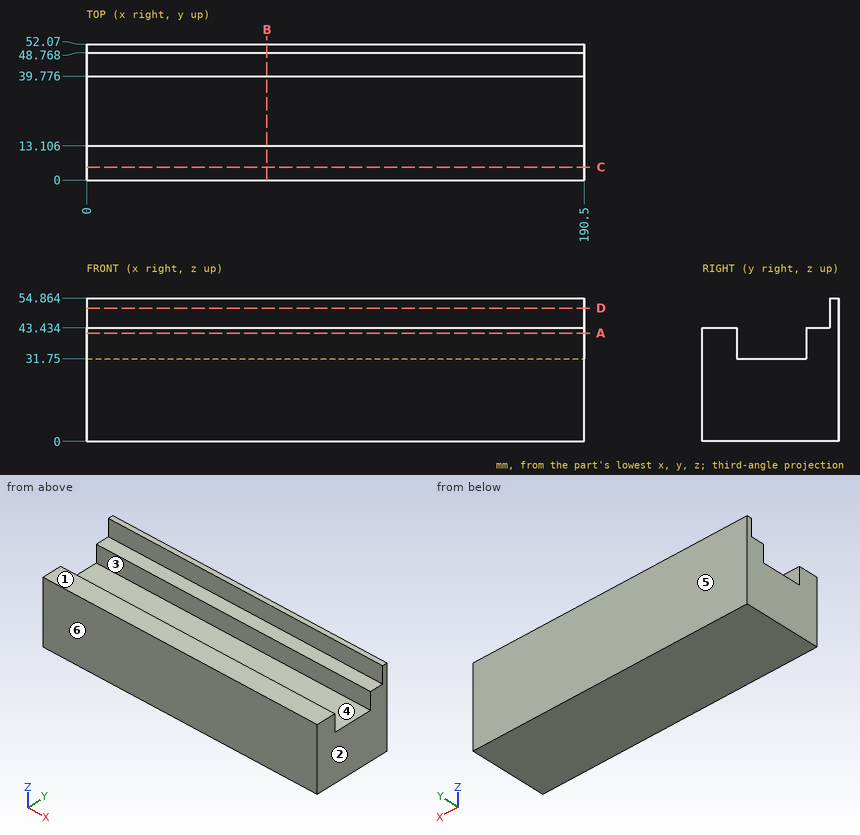
Geometry check sheet. Reference: drawing and pictorial views, mm from the part's lowest x, y, z. A direction names the side the tool comes from. Round coordinates to 2 decimals unless told otherwise and drop trailing zeros. Loops run counter-clockwise (first coordinate to the right, second up) from the corner with the lowest first, then second, coordinate; pieces in that order, holes last. Notation, with made-up numbers: M 36.25,50 L 86.25,50 A7 ccw 86.25,63 Z; hole C 81.5,1 d2. An arc over 180 degrees is marked long. Return JSON: item names as keys, results as strings. Group by question number.
(1) Section check C-C, the plane y = 5. Enter the section's corners in (x, z), and give its area (3 significant figures).
(2) Section check B-B, the plane x = 69. Enter the section's corners in (y, z).
(3) Section check A-A, the plane z = 41.5. Enter the section's corners in (x, y), and give its area (3 significant figures).
(4) Mould release check, pull along Y, two halves, no side actions. Record for the marked faces 4, 5 and 6: pulls with the +Y half, pulls with the -Y half, needs draft (parallel to the pull), parting line crosses it, or undercut.
(5) Section check D-D, the plane z = 51. Enter the section's corners in (x, y).
(6) Scan lines: line 1 along Y through (x, z) = (33, 39); line 2 along Y through (x, z) = (130.5, 48.5); line 3 along Z through (x, y) = (167.5, 9). Record each from-to range of solid material in increasing order. Write a range as [from, to].
(7) Set-up check for the marked faces 1, 2 and 3: record each of +Z, -Z, +X, -X, +Y, -Y from which the full face is reachable in a straight line by a thin tool's end or side.
(8) Go/stop test with flat-tipped pins: pin 1 (13.5 mm diameter, centred on x = 77, y = 22, fed in from +Z); pin 2 (14.5 mm diameter, centred on x = 137, y = 5.5, fed in from +Z); pin 3 (3 mm diameter, centred on y = 32, z = 34.5, fed in from +X); pin 4 (9 mm diameter, centred on x = 97, z = 49.5, fed in from -Y). Record where each tip stops, or that it passes through.
Data:
{
 "1": {"outline": "M 0,0 L 190.5,0 L 190.5,43.43 L 0,43.43 Z", "area": "8,270 mm²"},
 "2": {"outline": "M 0,0 L 52.07,0 L 52.07,54.86 L 48.77,54.86 L 48.77,43.43 L 39.78,43.43 L 39.78,31.75 L 13.11,31.75 L 13.11,43.43 L 0,43.43 Z"},
 "3": {"outline": "M 0,0 L 190.5,0 L 190.5,13.11 L 0,13.11 Z; M 0,39.78 L 190.5,39.78 L 190.5,52.07 L 0,52.07 Z", "area": "4,840 mm²"},
 "4": {"face 4": "undercut", "face 5": "pulls with the +Y half", "face 6": "pulls with the -Y half"},
 "5": {"outline": "M 0,48.77 L 190.5,48.77 L 190.5,52.07 L 0,52.07 Z"},
 "6": {"line 1": "[0, 13.11], [39.78, 52.07]", "line 2": "[48.77, 52.07]", "line 3": "[0, 43.43]"},
 "7": {"face 1": "+Z, +X, -X, -Y", "face 2": "+Z, -Z, +X, +Y, -Y", "face 3": "+Z, +X, -X"},
 "8": {"pin 1": "z = 31.75", "pin 2": "z = 43.43", "pin 3": "through", "pin 4": "y = 48.77"}
}
